The listing builds one solid part. Answer for the finished solid, in the listing's coordinates (mm). Coordinates: 2 decimals unless noted, no trailing zeros. Loops run counter-clockwise (first coordinate to the right, second up) from the corner with the lowest first, then second, coordinate; pieces in that order, holes last. Notation, with made-up numbers: (39, 58.5) - (54, 58.5) arc R27 ccw to (54, 89.5) - close; hole circle Ø6 at (87.5, 89.5). An arc over 180 degrees is marked (long way). Return JSON: item names as keys, results as strings. Group by question number.
1. Section A-A (y = -290) is taken. Write down the section's boundary in (x, z), and give its area (3 significant figures).
2. Each of these flat-tipped pins is pushed along its axis until it touches: P1, Ø8, axis at x = 23, y = -422.5, coming from the -Z side; P2, Ø4, axis at y = -319.5, z = 5, coming from the -X side; P3, Ø2, axis at y = -186, z = 5, coming from the +X side; P4, Ø11.5, axis at x = 23, y = -157.5, coming from the -Z side. Where does it stop, or does it pass through?
3. Section B-B (y = -447) is taken. Write down the section's boundary in (x, z), and give its area (3 significant figures).
4. Find the intervals of material crossed by line 1 along Y through (x, z) = (23, 18.5); line 2 along X through (y, z) = (-157.5, 22.75); line 3 along X through (y, z) = (-538, 23.25), in increasing order.
```python
from build123d import *

# Parameters (mm, degrees)
F1_DEPTH = 580
F2_R     = 5
F3_DEPTH = 20.001
F4_R     = 5


with BuildPart() as f1:
    # F0 (on Front) → F1 (new body)
    with BuildSketch(Plane.XZ):
        Polygon((0, 28), (0, 0), (15, 0), (15, 8), (31, 8), (31, 0), (50, 0), (60, 10), (60, 28), align=None)
    extrude(amount=F1_DEPTH)

    # F2 (on face) → F3 (cut, through all)
    with BuildSketch(Plane(origin=(0, 0, 8), x_dir=(1, 0, 0), z_dir=(0, 0, -1))):
        with Locations((23, 25)):
            Circle(F2_R)
        with Locations((23, 157.5)):
            Circle(F2_R)
        with Locations((23, 290)):
            Circle(F2_R)
        with Locations((23, 422.5)):
            Circle(F2_R)
        with Locations((23, 555)):
            Circle(F2_R)
    extrude(amount=-F3_DEPTH, mode=Mode.SUBTRACT)

    # F4
    f4_edges = [f1.edges().sort_by_distance(p)[0] for p in [
        (60, -290, 28),
    ]]
    fillet(f4_edges, radius=F4_R)


solid = f1.part
```
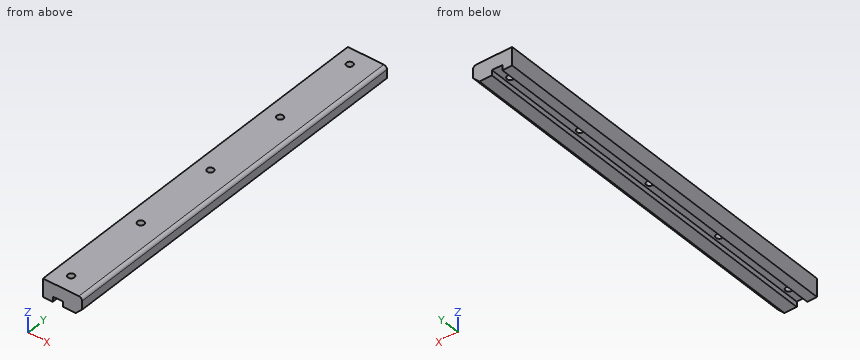
The answers:
{
 "1": {"outline": "(0, 0) - (15, 0) - (15, 8) - (18, 8) - (18, 28) - (0, 28) - close; (28, 8) - (31, 8) - (31, 0) - (50, 0) - (60, 10) - (60, 23) arc R5 ccw to (55, 28) - (28, 28) - close", "area": "1,300 mm2"},
 "2": {"P1": "passes through", "P2": "stops at x = 0", "P3": "stops at x = 56", "P4": "stops at z = 8"},
 "3": {"outline": "(0, 0) - (15, 0) - (15, 8) - (31, 8) - (31, 0) - (50, 0) - (60, 10) - (60, 23) arc R5 ccw to (55, 28) - (0, 28) - close", "area": "1,500 mm2"},
 "4": {"line 1": "y = -580 to -560, -550 to -427.5, -417.5 to -295, -285 to -162.5, -152.5 to -30, -20 to 0", "line 2": "x = 0 to 18, 28 to 60", "line 3": "x = 0 to 59.99"}
}
